Work out the finished part from the listing and answer in its coordinate system (mm). Face numbers are marked on the shaded views. A direction names the side the tool comes from. Coordinates: 2 decimals unless noted, no trailing zeros. Use a Markdown table: item, result. Add a question column.
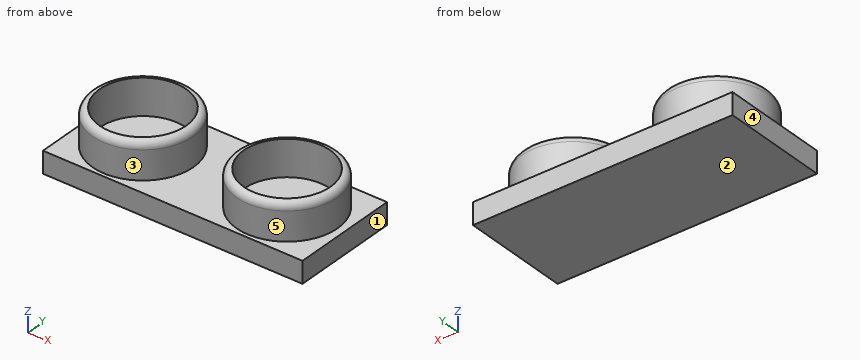
```python
from build123d import *

# Parameters (mm, degrees)
SKETCH1_W           = 36
SKETCH1_H           = 15
BOSS_EXTRUDE1_DEPTH = 3
SKETCH2_R           = 7
SKETCH2_R_2         = 6
BOSS_EXTRUDE2_DEPTH = 5
FILLET1_R           = 1


with BuildPart() as part:
    # Sketch1 → Boss-Extrude1 (new body)
    with BuildSketch(Plane.XY):
        Rectangle(SKETCH1_W, SKETCH1_H)
    extrude(amount=BOSS_EXTRUDE1_DEPTH)

    # Sketch2 → Boss-Extrude2 (add)
    # profile 1 of 2: a face of its own
    with BuildSketch(Plane.XY.offset(3)):
        with Locations((-10, 0)):
            Circle(SKETCH2_R)
        with Locations((-10, 0)):
            Circle(SKETCH2_R_2, mode=Mode.SUBTRACT)
    # profile 2 of 2: a face of its own
    with BuildSketch(Plane.XY.offset(3)):
        with Locations((10, 0)):
            Circle(SKETCH2_R)
        with Locations((10, 0)):
            Circle(SKETCH2_R_2, mode=Mode.SUBTRACT)
    extrude(amount=BOSS_EXTRUDE2_DEPTH)

    # Fillet1
    fillet1_edges = [part.edges().sort_by_distance(p)[0] for p in [
        (-17, 0, 8),
        (3, 0, 8),
    ]]
    fillet(fillet1_edges, radius=FILLET1_R - 0.0001)  # a hair under: the kernel refuses the full size


solid = part.part
```
Item 1: Given pin 1 (4 mm diameter, centred on x = -1, y = -2, fed in from -Z); pin 2 (2 mm diameter, centred on y = 3, z = 4.5, fed in from -X); pin 3 (1.5 mm diameter, centred on y = 2.5, z = 4, fed in from -X); pin 4 (3 mm diameter, centred on y = -5.5, z = 5.5, fed in from +X), each flat-ended and moving along its own axis, determine where each tip first touches the part or whether it passes through.
Item 2: For a pull along X with two mould halves and no side action, classify the marked faces 1, 2 and 3 as +X half, -X half, draft (parallel to the pull), parting line (faces both ways), or undercut.
Item 3: For the marked faces 4 and 5, determine the directions among +Z, -Z, +X, -X, +Y, -Y from which every point of the face is accessible in a straight line to the end or side of a thin tool.
Item 4: Find the intervals of material crossed by probe 1 along X at (y, z) = (-0.5, 6.5); probe 2 along Y at (x, z) = (-10, 6.15); probe 3 along X at (y, z) = (0.5, 7.25), in increasing order.
Output:
| question | item | result |
|---|---|---|
| 1 | pin 1 | stops at z = 0 |
| 1 | pin 2 | stops at x = -16.71 |
| 1 | pin 3 | stops at x = -16.78 |
| 1 | pin 4 | stops at x = 15.74 |
| 2 | face 1 | +X half |
| 2 | face 2 | draft |
| 2 | face 3 | undercut |
| 3 | face 4 | +Z, -Z, -X, +Y, -Y |
| 3 | face 5 | +Z |
| 4 | probe 1 | x = -16.98 to -15.98, -4.02 to -3.02, 3.02 to 4.02, 15.98 to 16.98 |
| 4 | probe 2 | y = -7 to -6, 6 to 7 |
| 4 | probe 3 | x = -16.95 to -15.98, -4.02 to -3.05, 3.05 to 4.02, 15.98 to 16.95 |
